Verification items for this drawing (mm, ordinates from the low corner). A direction names the side the tool comes from. Give positions to 0.01 mm unless a question says otherwise; leave off trailing zeros. Order: outer loops, then holes, each group sorted by start corner. A loop starts at its lowest first (then second) coordinate and runs counter-clockwise, first axis right, second up. Notation, with made-up numbers: M 35.5,32 L 49.5,32 A4 cw 49.5,39 Z; hole C 47,-37 d4. An arc over 180 degrees is marked long. Answer as a JSON object with one key per item and string values.
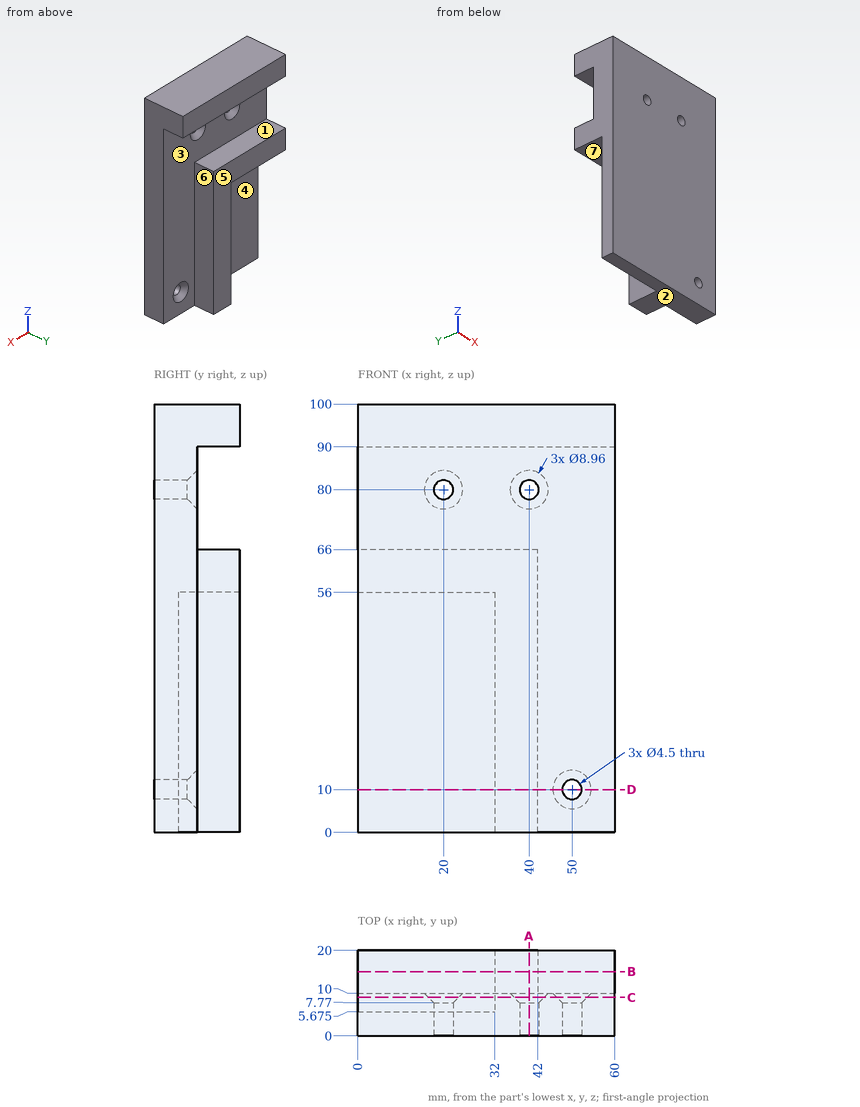
Q1. Section check D-D on z = 10. Record the cut outline in (x, y) (3 decimals), then the cut area to 3 significant figures.
Resolved:
{"outline": "M 0,0 L 47.75,0 L 47.75,7.77 L 45.52,10 L 42,10 L 42,20 L 32,20 L 32,5.675 L 0,5.675 Z; M 52.25,0 L 60,0 L 60,10 L 54.48,10 L 52.25,7.77 Z", "area": "512 mm²"}
Q2. Section check A-A on x = 40. Record the cut outline in (y, z), then the cut area to 3 significant figures.
Resolved:
{"outline": "M 0,0 L 20,0 L 20,66 L 10,66 L 10,75.52 L 7.77,77.75 L 0,77.75 Z; M 0,82.25 L 7.77,82.25 L 10,84.48 L 10,90 L 20,90 L 20,100 L 0,100 Z", "area": "1,710 mm²"}
Q3. Release check for a two-part mould opening along Z. For the marked faces 1, 2, 3 and 4 record: +Z half, -Z half, draft (parallel to the pull), parting line (faces both ways), or undercut.
Resolved:
{"face 1": "undercut", "face 2": "-Z half", "face 3": "undercut", "face 4": "draft"}
Q4. Section check B-B on y = 15. Record the cut outline in (x, z).
Resolved:
{"outline": "M 0,56 L 32,56 L 32,0 L 42,0 L 42,66 L 0,66 Z; M 0,90 L 60,90 L 60,100 L 0,100 Z"}
Q5. Material ranges on L1, parallel to X at y = 1.75, z = 80; L2, parallel to Z at x = 20, y = 7; L3, parallel to Z at x = 13, y = 19, recorded low to high.
Resolved:
{"L1": "x = 0 to 17.75, 22.25 to 37.75, 42.25 to 60", "L2": "z = 56 to 77.75, 82.25 to 100", "L3": "z = 56 to 66, 90 to 100"}
Q6. Gauge pin test, flat ends, axial feed: pin 1 Ø3 at (y, z) = (11.5, 12) entering from -X; pin 2 Ø4 at (x, z) = (20, 80) entering from -Y; pin 3 Ø7 at (x, y) = (11.5, 10.5) entering from -Z; pin 4 Ø4 at (x, z) = (9.5, 87) entering from +Y. Record the tip position at first contact, or that the pin passes through.
Resolved:
{"pin 1": "stops at x = 32", "pin 2": "passes through", "pin 3": "stops at z = 56", "pin 4": "stops at y = 10"}
Q7. Tool access check on the marked faces 5, 6 and 7. Record the directions out of +Z, -Z, +X, -X, +Y, -Y that give a thin tool (end or side, any length) a straight path to the whole face; none if there is none.
Resolved:
{"face 5": "+Z, -Z, +X, -X, +Y", "face 6": "-Z, +X, +Y", "face 7": "-Z, -X, +Y"}
Q8. Section check C-C on y = 9. Record the cut outline in (x, z), then the cut area to 3 significant figures.
Resolved:
{"outline": "M 0,56 L 32,56 L 32,0 L 60,0 L 60,100 L 0,100 Z; hole C 20,80 d6.96; hole C 40,80 d6.96; hole C 50,10 d6.96", "area": "4,090 mm²"}
